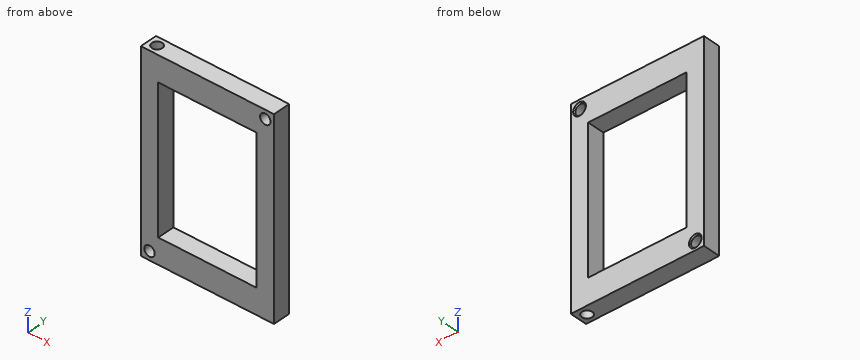
from build123d import *

# Parameters (mm, degrees)
BOSS_EXTRU_1_DEPTH      = 84
ESQUISSE3_R             = 2.25
ENL_V_MAT_EXTRU_1_DEPTH = 25
ENL_V_MAT_EXTRU_2_REACH = 9.5
ESQUISSE4_R             = 2.25
ESQUISSE4_W             = 42.5
ESQUISSE4_H             = 62.086956522
ESQUISSE5_R             = 2.25
ENL_V_MAT_EXTRU_3_DEPTH = 25
CHANFREIN1_SIZE         = 0.5


with BuildPart() as part:
    # Esquisse1 → Boss.-Extru.1 (new body)
    with BuildSketch(Plane.XY):
        Polygon((-15.842295968, 13.667406166), (-23.342295968, 13.667406166), (-23.342295968, 21.167406166), (34.157704032, 21.167406166), (34.157704032, 13.667406166), (26.657704032, 13.667406166), align=None)
    extrude(amount=BOSS_EXTRU_1_DEPTH)

    # Esquisse3 → Enlèv. mat.-Extru.1 (cut)
    with BuildSketch(Plane.XY.offset(84)):
        with Locations((-19.592295968, 17.417406166)):
            Circle(ESQUISSE3_R)
    extrude(amount=-ENL_V_MAT_EXTRU_1_DEPTH, mode=Mode.SUBTRACT)

    # Esquisse4 → Enlèv. mat.-Extru.2 (cut, up to next)
    with BuildSketch(Plane(origin=(0, 21.167406166, 0), x_dir=(1, 0, 0), z_dir=(0, 1, 0)), mode=Mode.PRIVATE) as enl_v_mat_extru_2_sk1:
        with Locations((30.407704032, -80.25)):
            Circle(ESQUISSE4_R)
    enl_v_mat_extru_2_tool1 = extrude(enl_v_mat_extru_2_sk1.sketch, amount=-ENL_V_MAT_EXTRU_2_REACH, mode=Mode.PRIVATE) & part.part
    add(enl_v_mat_extru_2_tool1.solids().sort_by_distance((30.407704, 21.167406, 80.25))[0], mode=Mode.SUBTRACT)
    # Esquisse4 → Enlèv. mat.-Extru.2 (cut, up to next)
    with BuildSketch(Plane(origin=(0, 21.167406166, 0), x_dir=(1, 0, 0), z_dir=(0, 1, 0)), mode=Mode.PRIVATE) as enl_v_mat_extru_2_sk2:
        with Locations((-19.592295968, -3.75)):
            Circle(ESQUISSE4_R)
    enl_v_mat_extru_2_tool2 = extrude(enl_v_mat_extru_2_sk2.sketch, amount=-ENL_V_MAT_EXTRU_2_REACH, mode=Mode.PRIVATE) & part.part
    add(enl_v_mat_extru_2_tool2.solids().sort_by_distance((-19.592296, 21.167406, 3.75))[0], mode=Mode.SUBTRACT)
    # Esquisse4 → Enlèv. mat.-Extru.2 (cut, up to next)
    with BuildSketch(Plane(origin=(0, 21.167406166, 0), x_dir=(1, 0, 0), z_dir=(0, 1, 0)), mode=Mode.PRIVATE) as enl_v_mat_extru_2_sk3:
        with Locations((5.407704032, -42)):
            Rectangle(ESQUISSE4_W, ESQUISSE4_H)
    enl_v_mat_extru_2_tool3 = extrude(enl_v_mat_extru_2_sk3.sketch, amount=-ENL_V_MAT_EXTRU_2_REACH, mode=Mode.PRIVATE) & part.part
    add(enl_v_mat_extru_2_tool3.solids().sort_by_distance((5.407704, 21.167406, 42))[0], mode=Mode.SUBTRACT)

    # Esquisse5 → Enlèv. mat.-Extru.3 (cut)
    with BuildSketch(Plane(origin=(0, 0, 0), x_dir=(-1, 0, 0), z_dir=(0, 0, -1))):
        with Locations((-30.407704032, 17.417406166)):
            Circle(ESQUISSE5_R)
    extrude(amount=-ENL_V_MAT_EXTRU_3_DEPTH, mode=Mode.SUBTRACT)

    # Chanfrein1
    chanfrein1_edges = [part.edges().sort_by_distance(p)[0] for p in [
        (28.157704032, 21.167406166, 80.25),
        (-21.842295968, 21.167406166, 3.75),
    ]]
    chamfer(chanfrein1_edges, length=CHANFREIN1_SIZE)


solid = part.part
Source: CAD feature listing. Evaluate the final solid. Frame: model axes, mm. Give positions to 0.01 mm unless a question says otherwise; leave off trailing zeros. Write each loop counter-clockwise with the first axis right and the second up, starting at its lowest first coordinate (ties: lowest second). Pieces come first, ordered by that corner, then holes. Notation, with made-up numbers: (58, 53) - (63, 53) arc R19 ccw to (63, 76) - close; hole circle Ø11 at (38.5, 60.25). An arc over 180 degrees is marked (long way). Write item = value, one per line. Start each with the question number.
Q1. Pin query (flat end, axial travel): pin 1 Ø2 at (x, y) = (30.5, 16.5) entering from -Z. Return the tip coordinate at first contact, or that it passes through.
Q2. Cut plane D-D, the plane z = 80.25. Return loops of the section in (x, y), then the cut area to 3 significant figures.
Q3. Cut plane C-C, the plane z = 41.5. Return loops of the section in (x, y), then the cut area to 4 significant figures.
Q4. Cut plane B-B, the plane z = 12.5. Return loops of the section in (x, y).
Q5. Cut plane A-A, the plane x = 16. Return loops of the section in (y, z).
Q6. Material intervals for probe 1 along Z at (x, y) = (6, 15); probe 2 along X at (y, z) = (18.5, 50.5); probe 3 along X at (y, z) = (17.5, 80), sorted ascending.
Computed values:
q1.pin_1 = 25
q2.outline = (-23.34, 13.67) - (28.16, 13.67) - (28.16, 20.67) - (27.66, 21.17) - (-23.34, 21.17) - close; (32.66, 13.67) - (34.16, 13.67) - (34.16, 21.17) - (33.16, 21.17) - (32.66, 20.67) - close; hole circle Ø4.5 at (-19.59, 17.42)
q2.area = 381 mm²
q3.outline = (-23.34, 13.67) - (-15.84, 13.67) - (-15.84, 21.17) - (-23.34, 21.17) - close; (26.66, 13.67) - (34.16, 13.67) - (34.16, 21.17) - (26.66, 21.17) - close
q3.area = 112.5 mm²
q4.outline = (-23.34, 13.67) - (-15.84, 13.67) - (-15.84, 21.17) - (-23.34, 21.17) - close; (26.66, 13.67) - (34.16, 13.67) - (34.16, 21.17) - (26.66, 21.17) - close; hole circle Ø4.5 at (30.41, 17.42)
q5.outline = (13.67, 0) - (21.17, 0) - (21.17, 10.96) - (13.67, 10.96) - close; (13.67, 73.04) - (21.17, 73.04) - (21.17, 84) - (13.67, 84) - close
q6.probe_1 = 0 to 10.96, 73.04 to 84
q6.probe_2 = -23.34 to -15.84, 26.66 to 34.16
q6.probe_3 = -23.34 to -21.84, -17.34 to 28.17, 32.64 to 34.16
